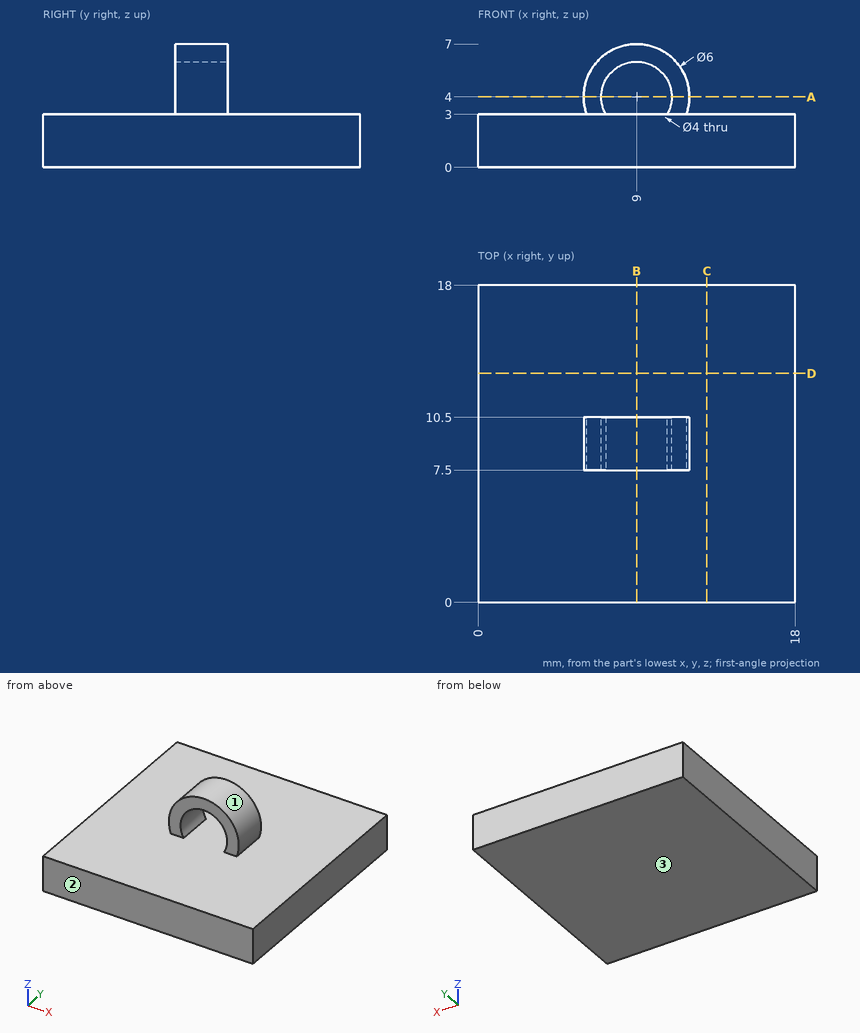
Answer from the drawing. Dimensions are ordinates in mm from the lowest x, y and z of the part. Give positions to 0.01 mm unless a question says otherwise; leave off trailing zeros. Loops run counter-clockwise (first coordinate to the right, second up) from the corner with the lowest first, then second, coordinate; pieces in that order, holes last.
Item 1: Find the intervals of material crossed by line 1 along X through (y, z) = (9.9, 4); line 2 along Z through (x, y) = (9, 9.45); line 3 along Z through (x, y) = (15.5, 3.25), in increasing order.
Item 2: The mould has two halves that part along Z. Classify the marked faces 1, 2 and 3: released by +Z, released by -Z, zero draft, split by the parting line, or undercut.
Item 3: The part is cut by section B-B (x = 9). Write down the section's boundary in (y, z), and give its area (3 significant figures).
Item 4: Each of these flat-tipped pins is pushed along its axis until it touches: pin 1 Ø1.5 at (x, z) = (15.5, 5) entering from -Y; pin 2 Ø1.2 at (x, z) = (10.5, 5) entering from +Y; pin 3 Ø2 at (x, y) = (15, 2.5) entering from +Z; pin 4 Ø1.2 at (x, z) = (8, 5.5) entering from -Y. Where does it stop, or does it pass through?
Item 5: The part is cut by section A-A (z = 4). Write down the section's boundary in (x, y).
Item 6: The part is cut by section C-C (x = 13). Write down the section's boundary in (y, z), and give its area (3 significant figures).
Taken from the geometry:
1. line 1: x = 6 to 7, 11 to 12
1. line 2: z = 0 to 3, 6 to 7
1. line 3: z = 0 to 3
2. face 1: undercut
2. face 2: zero draft
2. face 3: released by -Z
3. outline: (0, 0) - (18, 0) - (18, 3) - (0, 3) - close; (7.5, 6) - (10.5, 6) - (10.5, 7) - (7.5, 7) - close
3. area: 57.0 mm2
4. pin 1: passes through
4. pin 2: stops at y = 10.5
4. pin 3: stops at z = 3
4. pin 4: stops at y = 7.5
5. outline: (6, 7.5) - (7, 7.5) - (7, 10.5) - (6, 10.5) - close; (11, 7.5) - (12, 7.5) - (12, 10.5) - (11, 10.5) - close
6. outline: (0, 0) - (18, 0) - (18, 3) - (0, 3) - close
6. area: 54.0 mm2
